The listing builds one solid part. Answer for the finished solid, in the listing's coordinates (mm). Give positions to 0.01 mm unless a question says otherwise; leave off trailing zeros. Loops run counter-clockwise (first coordinate to the right, second up) from the corner with the lowest first, then second, coordinate; pieces in that order, holes last. Notation, with made-up numbers: (56, -19.5) - (67, -19.5) arc R24 ccw to (67, 4.5) - close; hole circle Ø11 at (-34, -13). An arc over 180 degrees is marked (long way). Write item = value, one per line. Start each with the question number.
1) The part is cut by section B-B on z = 0.4. Write down the section's boundary in (x, y), plus the area to 3 significant figures.
2) The part is cut by section A-A on y = 40.5. Write down the section's boundary in (x, z), plus the area to 3 significant figures.
3) Flat-ended cylindrical pins translate along their axes: P1, Ø0.6, axis at y = 16, z = 0.5, coming from the +X side; P2, Ø6.5, axis at x = 45.24, y = 40.5, coming from the +Z side. Find the tip coordinate at first contact, or state that the pin passes through.
4) The part is cut by section C-C on x = -74. Write down the section's boundary in (y, z), plus the area to 3 significant figures.
5) Consider probe 1 along X at (y, z) = (40.5, 0.9); probe 2 along Y at (x, z) = (-87, 1.15); probe 3 along Y at (x, z) = (-187.5, 0.5). Determine where each line is inside the solid, lowest interval first.
6) The part is cut by section D-D on y = 24. Write down the section's boundary in (x, z), plus the area to 3 significant figures.
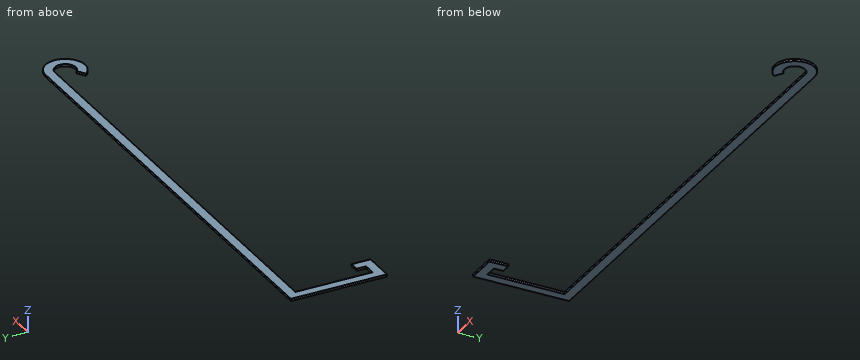
from build123d import *

# Parameters (mm, degrees)
F1_DEPTH = 1.2


with BuildPart() as f1:
    # F0 (on Top) → F1 (new body)
    with BuildSketch(Plane.XY):
        with BuildLine():
            Line((-201.25569, 51), (-201.25569, 0))
            Line((-201.25569, 0), (-184.75569, 0))
            Line((-184.75569, 0), (-184.75569, 10))
            Line((-184.75569, 10), (-189.75569, 10))
            Line((-189.75569, 10), (-189.75569, 5))
            Line((-189.75569, 5), (-196.25569, 5))
            Line((-196.25569, 5), (-196.25569, 46))
            Line((-196.25569, 46), (-184.75569, 46))
            Line((-184.75569, 46), (45.24431, 46))
            ThreePointArc((45.24431, 46), (50.378713, 38.528222), (41.562891, 36.413785))
            Line((41.562891, 36.413785), (37.243051, 33.700747))
            ThreePointArc((37.243051, 33.700747), (54.77432, 36.092175), (45.24431, 51))
            Line((45.24431, 51), (-184.75569, 51))
            Line((-184.75569, 51), (-201.25569, 51))
        make_face()
    extrude(amount=F1_DEPTH)


solid = f1.part
Answer below:
q1.outline = (-201.26, 0) - (-184.76, 0) - (-184.76, 10) - (-189.76, 10) - (-189.76, 5) - (-196.26, 5) - (-196.26, 46) - (45.24, 46) arc R5.5 cw (long way) to (41.56, 36.41) - (37.24, 33.7) arc R10.5 ccw (long way) to (45.24, 51) - (-201.26, 51) - close
q1.area = 1,700 mm2
q2.outline = (-201.26, 0) - (-196.26, 0) - (-196.26, 1.2) - (-201.26, 1.2) - close; (50.74, 0) - (55.74, 0) - (55.74, 1.2) - (50.74, 1.2) - close
q2.area = 12.0 mm2
q3.P1 = -196.26
q3.P2 = through
q4.outline = (46, 0) - (51, 0) - (51, 1.2) - (46, 1.2) - close
q4.area = 6.00 mm2
q5.probe_1 = -201.26 to -196.26, 50.74 to 55.74
q5.probe_2 = 46 to 51
q5.probe_3 = 0 to 10, 46 to 51
q6.outline = (-201.26, 0) - (-196.26, 0) - (-196.26, 1.2) - (-201.26, 1.2) - close
q6.area = 6.00 mm2
